Source: CAD feature listing. Evaluate the final solid. Frame: model axes, mm. Face numbers are marked on the shaded views. A direction names the side the tool comes from. Give positions to 0.01 mm unless a question says otherwise; leave off trailing zeros. Loops run counter-clockwise (first coordinate to the right, second up) from the corner with the lowest first, then second, coordinate; pieces in that order, holes last. Notation, with made-up numbers: (14, 35) -> (50, 35) arc R36 ccw to (50, 74) -> close; hole circle Ø9 at (22.5, 4.5). An arc over 180 degrees is marked (long way). Return JSON: item names as keys, results as strings. Group by question number.
(1) Access query for the marked faces 1 and 2. Directions: +Z, -Z, +X, -X, +Y, -Y. A direction counts if a zero-diameter tool reaches every point of the face in a straight line with its end or side. Return the directions, or none.
(2) Ray query, line 1 (Z direction, x = 77.5, y = 22); line 2 (Y direction, x = 104, z = 126.5); line 3 (Y direction, x = 80, z = 95). Return the intervals inside material, ascending. Write a range as from..to.
(3) Cut plane C-C on z = 122. Return loops of the section in (x, y).
(4) Draft query along X for the marked faces 3, 4, 5 and 6. Return one class per face: released by +X, released by -X, zero draft, split by the parting line, or undercut.
(5) Cut plane D-D on z = 87.5. Return loops of the section in (x, y), then the cut area to 3 significant figures.
(6) Pin query (flat end, axial travel): pin 1 (6 mm diameter, centred on x = 88, z = 71, fed in from +Y); pin 2 (1.5 mm diameter, centred on y = 108.5, z = 54.5, fed in from -X); pin 3 (1 mm diameter, centred on x = 93, z = 98.5, fed in from -Y). Return the tip coordinate at first contact, or that it passes through.
```python
from build123d import *

# Parameters (mm, degrees)
SKETCH1_W               = 160
SKETCH1_H               = 160
BOSS_EXTRUDE1_DEPTH     = 30
SKETCH2_W               = 140
SKETCH2_H               = 140
BOSS_EXTRUDE2_DEPTH     = 80
BOSS_EXTRUDE2_TAPER     = 5
SKETCH3_R               = 40
BOSS_EXTRUDE3_DEPTH     = 30
CUT_EXTRUDE1_DEPTH      = 267.082693913
CUT_EXTRUDE1_DEPTH_BACK = 267.082693913
SKETCH4_R               = 30
FILLET1_R               = 5
CHAMFER1_SIZE           = 10


with BuildPart() as part:
    # Sketch1 → Boss-Extrude1 (new body)
    with BuildSketch(Plane.XY):
        with Locations((80, 80)):
            Rectangle(SKETCH1_W, SKETCH1_H)
    extrude(amount=BOSS_EXTRUDE1_DEPTH)

    # Sketch2 → Boss-Extrude2 (add)
    with BuildSketch(Plane.XY.offset(30)):
        with Locations((80, 80)):
            Rectangle(SKETCH2_W, SKETCH2_H)
    extrude(amount=BOSS_EXTRUDE2_DEPTH, taper=BOSS_EXTRUDE2_TAPER)

    # Sketch3 → Boss-Extrude3 (add)
    with BuildSketch(Plane.XY.offset(110)):
        with Locations((80, 80)):
            Circle(SKETCH3_R)
    extrude(amount=BOSS_EXTRUDE3_DEPTH)

    # Sketch4 → Cut-Extrude1 (cut, two sides: drawn at the far end of the back side and taken through both)
    with BuildSketch(Plane.XY.offset(140).offset(-CUT_EXTRUDE1_DEPTH_BACK)):
        with Locations((80, 80)):
            Circle(SKETCH4_R)
    extrude(amount=CUT_EXTRUDE1_DEPTH + CUT_EXTRUDE1_DEPTH_BACK, mode=Mode.SUBTRACT)

    # Fillet1
    fillet1_edges = [part.edges().sort_by_distance(p)[0] for p in [
        (16.999093082, 80, 110),
        (80, 16.999093082, 110),
        (143.000906918, 80, 110),
        (80, 143.000906918, 110),
        (40, 80, 110),
    ]]
    fillet(fillet1_edges, radius=FILLET1_R)

    # Chamfer1
    chamfer1_edges = [part.edges().sort_by_distance(p)[0] for p in [
        (160, 80, 30),
        (80, 160, 30),
        (0, 80, 30),
        (80, 0, 30),
    ]]
    chamfer(chamfer1_edges, length=CHAMFER1_SIZE - 0.0001)  # a hair under: the kernel refuses the full size


solid = part.part
```
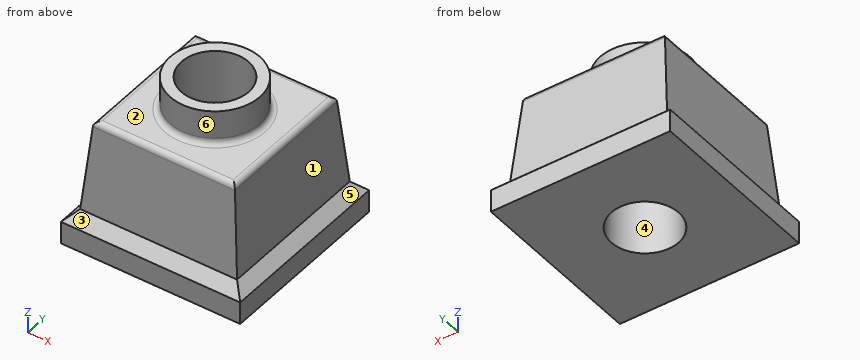
Answers:
{
 "1": {"face 1": "+Z, +X, +Y, -Y", "face 2": "+Z"},
 "2": {"line 1": "0..110", "line 2": "48..62, 98..112", "line 3": "15.69..50, 110..144.31"},
 "3": {"outline": "circle Ø80 at (80, 80); hole circle Ø60 at (80, 80)"},
 "4": {"face 3": "zero draft", "face 4": "undercut", "face 5": "released by +X", "face 6": "split by the parting line"},
 "5": {"outline": "(15.03, 15.03) -> (144.97, 15.03) -> (144.97, 144.97) -> (15.03, 144.97) -> close; hole circle Ø60 at (80, 80)", "area": "14,100 mm²"},
 "6": {"pin 1": "y = 146.68", "pin 2": "x = 12.08", "pin 3": "y = 15.95"}
}
